CAD build for the part. Positions are in the model's coordinates, mm. A direction names the side the tool comes from. Coordinates: 2 decimals unless noted, no trailing zeros. Order: outer loops, then holes, each group sorted by start corner. A loop starts at its lowest first (then second) coordinate and runs counter-clockwise, first axis right, second up. Notation, with made-up numbers: M 89.5,33.25 L 104.5,33.25 A22 cw 104.5,56.25 Z; hole C 83,32.5 d9. An arc over 180 degrees is marked long. Write item = value, one per line.
from build123d import *

# Parameters (mm, degrees)
SKETCH1_W           = 101.6
SKETCH1_H           = 50.8
SKETCH1_R           = 10.5
SKETCH1_R_2         = 1.5
BOSS_EXTRUDE1_DEPTH = 6.35
SKETCH2_R           = 21
CUT_EXTRUDE1_DEPTH  = 3.175
SKETCH3_R           = 3.25
CUT_EXTRUDE2_DEPTH  = 7.35
FILLET1_R           = 10


with BuildPart() as part:
    # Sketch1 → Boss-Extrude1 (new body)
    with BuildSketch(Plane.XY):
        with Locations((0, -0.237458689)):
            Rectangle(SKETCH1_W, SKETCH1_H)
        with Locations((0, -0.237458689)):
            Circle(SKETCH1_R, mode=Mode.SUBTRACT)
        with Locations((-9.72, 9.482541311)):
            Circle(SKETCH1_R_2, mode=Mode.SUBTRACT)
        with Locations((9.72, 9.482541311)):
            Circle(SKETCH1_R_2, mode=Mode.SUBTRACT)
        with Locations((9.72, -9.957458689)):
            Circle(SKETCH1_R_2, mode=Mode.SUBTRACT)
        with Locations((-9.72, -9.957458689)):
            Circle(SKETCH1_R_2, mode=Mode.SUBTRACT)
    extrude(amount=BOSS_EXTRUDE1_DEPTH)

    # Sketch2 → Cut-Extrude1 (cut)
    with BuildSketch(Plane(origin=(0, 0, 0), x_dir=(-1, 0, 0), z_dir=(0, 0, -1))):
        Circle(SKETCH2_R)
    extrude(amount=-CUT_EXTRUDE1_DEPTH, mode=Mode.SUBTRACT)

    # Sketch3 → Cut-Extrude2 (cut, through all)
    with BuildSketch(Plane.XY.offset(6.35)):
        with Locations((-38.1, -0.237458689)):
            Circle(SKETCH3_R)
        with Locations((38.1, -0.237458689)):
            Circle(SKETCH3_R)
    extrude(amount=-CUT_EXTRUDE2_DEPTH, mode=Mode.SUBTRACT)

    # Fillet1
    fillet1_edges = [part.edges().sort_by_distance(p)[0] for p in [
        (50.8, -25.637458689, 3.175),
        (-50.8, -25.637458689, 3.175),
        (-50.8, 25.162541311, 3.175),
        (50.8, 25.162541311, 3.175),
    ]]
    fillet(fillet1_edges, radius=FILLET1_R)


solid = part.part
(1) Tool access for faces 1 (the face through (-4, 10, 3.175)), 2 (the face through (-11.22, 9.55, 4.74)): list every direction of +Z, -Z, +X, -X, +Y, -Y with a clear straight run to the whole face (end or side of a thin tool).
Evaluation:
face_1 = -Z
face_2 = +Z, -Z
(2) Wall check: line 1 (Z direction, x = 3, y = 19) (3 decimals); line 2 (Y direction, x = 13.5, z = 0.75); line 3 (Y direction, x = 39, z = 6). Give the ranges that are in metal, low to high. Write a range as from..to.
Evaluation:
line_1 = 3.175..6.35
line_2 = -25.64..-16.09, 16.09..25.16
line_3 = -25.64..-3.36, 2.89..25.16
(3) Slice it at A-A, the plane x = 0. Write the cut outline in (y, z) (3 decimals), then the cut area to 3 significant figures.
Evaluation:
outline = M -25.637,0 L -21,0 L -21,3.175 L -10.737,3.175 L -10.737,6.35 L -25.637,6.35 Z; M 10.263,3.175 L 21,3.175 L 21,0 L 25.163,0 L 25.163,6.35 L 10.263,6.35 Z
area = 123 mm²
(4) Slice it at C-C, the plane z = 1.5. Write the cut outline in (x, y).
Evaluation:
outline = M -50.8,-15.64 A10 ccw -40.8,-25.64 L 40.8,-25.64 A10 ccw 50.8,-15.64 L 50.8,15.16 A10 ccw 40.8,25.16 L -40.8,25.16 A10 ccw -50.8,15.16 Z; hole C -38.1,-0.24 d6.5; hole C 0,0 d42; hole C 38.1,-0.24 d6.5
(5) Slice it at D-D, the plane x = -38.1. Write the cut outline in (y, z).
Evaluation:
outline = M -25.64,0 L -3.49,0 L -3.49,6.35 L -25.64,6.35 Z; M 3.01,0 L 25.16,0 L 25.16,6.35 L 3.01,6.35 Z
(6) Slice it at B-B, the plane y = 6. Write the cut outline in (x, z) (3 decimals), then the cut area to 3 significant figures.
Evaluation:
outline = M -50.8,0 L -20.125,0 L -20.125,3.175 L -8.447,3.175 L -8.447,6.35 L -50.8,6.35 Z; M 8.447,3.175 L 20.125,3.175 L 20.125,0 L 50.8,0 L 50.8,6.35 L 8.447,6.35 Z
area = 464 mm²
(7) Pin check, flat tips, straight feed: pin 1 Ø2.5 at (x, y) = (-9.72, 9.48) entering from -Z; pin 2 Ø12.5 at (x, y) = (8, 1.5) entering from -Z (3 decimals). Stop position of each tip, or through.
Evaluation:
pin_1 = through
pin_2 = 3.175
